from build123d import *

# Parameters (mm, degrees)
SKETCH2_W            = 230
SKETCH2_H            = 42
BOSS_EXTRUDE1_DEPTH  = 60
BOSS_EXTRUDE2_DEPTH  = 150
SKETCH5_R            = 4
CUT_EXTRUDE1_DEPTH   = 277
SKETCH7_R            = 4
BOSS_EXTRUDE3_DEPTH  = 20
SKETCH7_2_R          = 4
CUT_EXTRUDE2_DEPTH   = 10
SKETCH8_W            = 62
SKETCH8_H            = 24.6
BOSS_EXTRUDE4_DEPTH  = 14
SKETCH9_W            = 62
SKETCH9_H            = 24.6
BOSS_EXTRUDE5_DEPTH  = 14
SKETCH15_W           = 42
SKETCH15_H           = 60
SKETCH15_R           = 4
CUT_EXTRUDE3_DEPTH   = 5
SKETCH17_W           = 42
SKETCH17_H           = 60
SKETCH17_R           = 4
CUT_EXTRUDE4_DEPTH   = 5
SKETCH18_W           = 1
SKETCH18_H           = 62
BOSS_EXTRUDE9_DEPTH  = 24.6
SKETCH18_3_R         = 3
CUT_EXTRUDE5_DEPTH   = 35
SKETCH19_W           = 1
SKETCH19_H           = 62
BOSS_EXTRUDE10_DEPTH = 24.6
SKETCH19_3_R         = 3
CUT_EXTRUDE6_DEPTH   = 27
SKETCH20_W           = 15
SKETCH20_H           = 62
SKETCH20_R           = 3
BOSS_EXTRUDE11_DEPTH = 1
SKETCH21_W           = 15
SKETCH21_H           = 62
SKETCH21_R           = 3
BOSS_EXTRUDE12_DEPTH = 1
SKETCH23_W           = 255
SKETCH23_H           = 10
BOSS_EXTRUDE13_DEPTH = 150
SKETCH25_W           = 251.390716306
SKETCH25_H           = 22.262694164
CUT_EXTRUDE7_DEPTH   = 150
BOSS_EXTRUDE16_DEPTH = 17
CUT_EXTRUDE8_DEPTH   = 150
SKETCH28_W           = 255
SKETCH28_H           = 13
CUT_EXTRUDE9_DEPTH   = 167
BOSS_EXTRUDE18_DEPTH = 6
CUT_EXTRUDE10_DEPTH  = 43
SKETCH32_W           = 10
SKETCH32_H           = 20
BOSS_EXTRUDE19_DEPTH = 7.5
SKETCH33_W           = 10
SKETCH33_H           = 20
BOSS_EXTRUDE20_DEPTH = 8
SKETCH38_R           = 2.5
CUT_EXTRUDE12_DEPTH  = 16
SKETCH40_W           = 20.026518065
SKETCH40_H           = 12.666252083
CUT_EXTRUDE13_DEPTH  = 116
SKETCH41_W           = 84.423481935
SKETCH41_H           = 10
SKETCH41_W_2         = 110.05
BOSS_EXTRUDE21_DEPTH = 61.47
SKETCH42_W           = 10
SKETCH42_H           = 25
CUT_EXTRUDE14_DEPTH  = 10
SKETCH40_3_W         = 20
SKETCH40_3_H         = 10
BOSS_EXTRUDE22_DEPTH = 162.1
SKETCH43_W           = 10
SKETCH43_H           = 31.300449652
BOSS_EXTRUDE23_DEPTH = 40.5
BOSS_EXTRUDE24_START = -60
SKETCH46_W           = 20
SKETCH46_H           = 20
BOSS_EXTRUDE24_DEPTH = 222.1
SKETCH48_R           = 2
CUT_EXTRUDE15_DEPTH  = 30


with BuildPart() as part:
    # Sketch2 → Boss-Extrude1 (new body)
    with BuildSketch(Plane(origin=(0, 0, 0), x_dir=(1, 0, 0), z_dir=(0, 1, 0))):
        Polygon((-125, -31), (125, -31), (125, -21), (125, 0), (125, 21), (125, 31), (-125, 31), (-125, 21), (-125, 0), (-125, -21), align=None)
        Rectangle(SKETCH2_W, SKETCH2_H, mode=Mode.SUBTRACT)
    extrude(amount=BOSS_EXTRUDE1_DEPTH)

    # Sketch4 → Boss-Extrude2 (add)
    with BuildSketch(Plane.XZ):
        Polygon((125, 31), (-125, 31), (-125, 21), (-115, 21), (125, 21), align=None)
    extrude(amount=BOSS_EXTRUDE2_DEPTH)

    # Sketch5 → Cut-Extrude1 (cut)
    with BuildSketch(Plane.ZY.offset(125)):
        with Locations((0, 15.395589143)):
            Circle(SKETCH5_R)
        with Locations((0, 45.395589143)):
            Circle(SKETCH5_R)
    extrude(amount=-CUT_EXTRUDE1_DEPTH, mode=Mode.SUBTRACT)

    # Sketch7 → Boss-Extrude3 (add)
    with BuildSketch(Plane(origin=(125, 0, 0), x_dir=(0, 0, -1), z_dir=(1, 0, 0))):
        Polygon((-21, -150), (-31, -150), (-31, 60), (31, 60), (31, 0), (-21, 0), align=None)
        with Locations((0, 15.395589143)):
            Circle(SKETCH7_R, mode=Mode.SUBTRACT)
        with Locations((0, 45.395589143)):
            Circle(SKETCH7_R, mode=Mode.SUBTRACT)
    extrude(amount=-BOSS_EXTRUDE3_DEPTH)

    # Sketch7<2> → Cut-Extrude2 (cut)
    with BuildSketch(Plane(origin=(125, 0, 0), x_dir=(0, 0, -1), z_dir=(1, 0, 0))):
        Polygon((-21, -150), (-31, -150), (-31, 60), (31, 60), (31, 0), (-21, 0), align=None)
        with Locations((0, 15.395589143)):
            Circle(SKETCH7_2_R, mode=Mode.SUBTRACT)
        with Locations((0, 45.395589143)):
            Circle(SKETCH7_2_R, mode=Mode.SUBTRACT)
    extrude(amount=-CUT_EXTRUDE2_DEPTH, mode=Mode.SUBTRACT)

    # Sketch8 → Boss-Extrude4 (add)
    with BuildSketch(Plane(origin=(115, 0, 0), x_dir=(0, 0, -1), z_dir=(1, 0, 0))):
        with Locations((0, 12.3)):
            Rectangle(SKETCH8_W, SKETCH8_H)
    extrude(amount=BOSS_EXTRUDE4_DEPTH)

    # Sketch9 → Boss-Extrude5 (add)
    with BuildSketch(Plane.ZY.offset(125)):
        with Locations((0, 47.7)):
            Rectangle(SKETCH9_W, SKETCH9_H)
    extrude(amount=BOSS_EXTRUDE5_DEPTH)

    # Sketch15 → Cut-Extrude3 (cut)
    with BuildSketch(Plane.ZY.offset(-105)):
        with Locations((0, 30)):
            Rectangle(SKETCH15_W, SKETCH15_H)
        with Locations((0, 15.395589143)):
            Circle(SKETCH15_R, mode=Mode.SUBTRACT)
        with Locations((0, 45.395589143)):
            Circle(SKETCH15_R, mode=Mode.SUBTRACT)
    extrude(amount=-CUT_EXTRUDE3_DEPTH, mode=Mode.SUBTRACT)

    # Sketch17 → Cut-Extrude4 (cut)
    with BuildSketch(Plane(origin=(-115, 0, 0), x_dir=(0, 0, -1), z_dir=(1, 0, 0))):
        with Locations((0, 30)):
            Rectangle(SKETCH17_W, SKETCH17_H)
        with Locations((0, 45.395589143)):
            Circle(SKETCH17_R, mode=Mode.SUBTRACT)
        with Locations((0, 15.395589143)):
            Circle(SKETCH17_R, mode=Mode.SUBTRACT)
    extrude(amount=-CUT_EXTRUDE4_DEPTH, mode=Mode.SUBTRACT)

    # Sketch18 → Boss-Extrude9 (add)
    with BuildSketch(Plane.XZ.offset(-35.4)):
        with Locations((-139.5, 0)):
            Rectangle(SKETCH18_W, SKETCH18_H)
    extrude(amount=-BOSS_EXTRUDE9_DEPTH)

    # Sketch18<3> → Cut-Extrude5 (cut)
    with BuildSketch(Plane.XZ.offset(-35.4)):
        with Locations((-132.5, 21)):
            Circle(SKETCH18_3_R)
        with Locations((-132.5, -21)):
            Circle(SKETCH18_3_R)
    extrude(amount=-CUT_EXTRUDE5_DEPTH, mode=Mode.SUBTRACT)

    # Sketch19 → Boss-Extrude10 (add)
    with BuildSketch(Plane(origin=(0, 24.6, 0), x_dir=(1, 0, 0), z_dir=(0, 1, 0))):
        with Locations((129.5, 0)):
            Rectangle(SKETCH19_W, SKETCH19_H)
    extrude(amount=-BOSS_EXTRUDE10_DEPTH)

    # Sketch19<3> → Cut-Extrude6 (cut)
    with BuildSketch(Plane(origin=(0, 24.6, 0), x_dir=(1, 0, 0), z_dir=(0, 1, 0))):
        with Locations((122.5, 21)):
            Circle(SKETCH19_3_R)
        with Locations((122.5, -21)):
            Circle(SKETCH19_3_R)
    extrude(amount=-CUT_EXTRUDE6_DEPTH, mode=Mode.SUBTRACT)

    # Sketch20 → Boss-Extrude11 (add)
    with BuildSketch(Plane(origin=(0, 24.6, 0), x_dir=(1, 0, 0), z_dir=(0, 1, 0))):
        with Locations((122.5, 0)):
            Rectangle(SKETCH20_W, SKETCH20_H)
        with Locations((122.5, -21)):
            Circle(SKETCH20_R, mode=Mode.SUBTRACT)
        with Locations((122.5, 21)):
            Circle(SKETCH20_R, mode=Mode.SUBTRACT)
    extrude(amount=BOSS_EXTRUDE11_DEPTH)

    # Sketch21 → Boss-Extrude12 (add)
    with BuildSketch(Plane.XZ.offset(-35.4)):
        with Locations((-132.5, 0)):
            Rectangle(SKETCH21_W, SKETCH21_H)
        with Locations((-132.5, 21)):
            Circle(SKETCH21_R, mode=Mode.SUBTRACT)
        with Locations((-132.5, -21)):
            Circle(SKETCH21_R, mode=Mode.SUBTRACT)
    extrude(amount=BOSS_EXTRUDE12_DEPTH)

    # Sketch23 → Boss-Extrude13 (add)
    with BuildSketch(Plane.XZ):
        with Locations((2.5, -26)):
            Rectangle(SKETCH23_W, SKETCH23_H)
    extrude(amount=BOSS_EXTRUDE13_DEPTH)

    # Sketch25 → Cut-Extrude7 (cut)
    with BuildSketch(Plane.XZ):
        with Locations((-4.583562675, 27.327499947)):
            Rectangle(SKETCH25_W, SKETCH25_H)
    extrude(amount=CUT_EXTRUDE7_DEPTH, mode=Mode.SUBTRACT)

    # Sketch26 → Boss-Extrude16 (add)
    with BuildSketch(Plane(origin=(0, 0, -31), x_dir=(-1, 0, 0), z_dir=(0, 0, -1))):
        Polygon((125, -150), (-130, -150), (-130, 25.6), (-115, 25.6), (-115, 60), (125, 60), (140, 60), (140, 34.4), (125, 34.4), (125, 25.6), align=None)
    extrude(amount=BOSS_EXTRUDE16_DEPTH)

    # Sketch27 → Cut-Extrude8 (cut)
    with BuildSketch(Plane.XZ):
        Polygon((110, -31), (132.347433228, -31), (132.347433228, -21), (110, -21), (-153.412168614, -21), (-153.412168614, -31), align=None)
    extrude(amount=CUT_EXTRUDE8_DEPTH, mode=Mode.SUBTRACT)

    # Sketch28 → Cut-Extrude9 (cut)
    with BuildSketch(Plane.XZ):
        with Locations((2.5, -37.5)):
            Rectangle(SKETCH28_W, SKETCH28_H)
    extrude(amount=CUT_EXTRUDE9_DEPTH, mode=Mode.SUBTRACT)

    # Sketch29 → Boss-Extrude18 (add)
    with BuildSketch(Plane(origin=(0, 0, -48), x_dir=(-1, 0, 0), z_dir=(0, 0, -1))):
        Polygon((125, -150), (-130, -150), (-130, 25.6), (-115, 25.6), (-115, 60), (125, 60), (140, 60), (140, 34.4), (125, 34.4), (125, 25.6), align=None)
    extrude(amount=BOSS_EXTRUDE18_DEPTH)

    # Sketch31 → Cut-Extrude10 (cut)
    with BuildSketch(Plane.XY.offset(-44)):
        Polygon((33.05, -150), (130, -150), (130, -100.63), (33.05, -100.63), (33.05, -80.63), (-22.95, -80.63), (-22.95, -100.63), (-125, -100.63), (-125, -150), align=None)
    extrude(amount=-CUT_EXTRUDE10_DEPTH, mode=Mode.SUBTRACT)

    # Sketch32 → Boss-Extrude19 (add)
    with BuildSketch(Plane.ZY.offset(-33.05)):
        with Locations((-49, -90.63)):
            Rectangle(SKETCH32_W, SKETCH32_H)
    extrude(amount=BOSS_EXTRUDE19_DEPTH)

    # Sketch33 → Boss-Extrude20 (add)
    with BuildSketch(Plane(origin=(-22.95, 0, 0), x_dir=(0, 0, -1), z_dir=(1, 0, 0))):
        with Locations((49, -90.63)):
            Rectangle(SKETCH33_W, SKETCH33_H)
    extrude(amount=BOSS_EXTRUDE20_DEPTH)

    # Sketch38 → Cut-Extrude12 (cut)
    with BuildSketch(Plane.XY.offset(-44)):
        with Locations((29.35, -95.53)):
            Circle(SKETCH38_R)
        with Locations((29.35, -85.73)):
            Circle(SKETCH38_R)
        with Locations((-19.25, -95.53)):
            Circle(SKETCH38_R)
        with Locations((-19.25, -85.73)):
            Circle(SKETCH38_R)
    extrude(amount=-CUT_EXTRUDE12_DEPTH, mode=Mode.SUBTRACT)

    # Sketch40 → Cut-Extrude13 (cut)
    with BuildSketch(Plane.XZ):
        with Locations((119.986740967, -50.333126042)):
            Rectangle(SKETCH40_W, SKETCH40_H)
    extrude(amount=CUT_EXTRUDE13_DEPTH, mode=Mode.SUBTRACT)

    # Sketch41 → Boss-Extrude21 (add)
    with BuildSketch(Plane.XZ.offset(100.63)):
        with Locations((67.761740968, -49)):
            Rectangle(SKETCH41_W, SKETCH41_H)
        with Locations((-69.975, -49)):
            Rectangle(SKETCH41_W_2, SKETCH41_H)
    extrude(amount=BOSS_EXTRUDE21_DEPTH)

    # Sketch42 → Cut-Extrude14 (cut)
    with BuildSketch(Plane.ZY.offset(-25.55)):
        with Locations((-49, -118.299550348)):
            Rectangle(SKETCH42_W, SKETCH42_H)
    cut_extrude14 = extrude(amount=-CUT_EXTRUDE14_DEPTH, mode=Mode.SUBTRACT)

    # Mirror1: Cut-Extrude14 across plane
    add(cut_extrude14.mirror(Plane.ZY.offset(-5.3)), mode=Mode.SUBTRACT)

    # Sketch40<3> → Boss-Extrude22 (add)
    with BuildSketch(Plane.XZ):
        with Locations((79.973481935, -39)):
            Rectangle(SKETCH40_3_W, SKETCH40_3_H)
        with Locations((-89.973481935, -39)):
            Rectangle(SKETCH40_3_W, SKETCH40_3_H)
    extrude(amount=BOSS_EXTRUDE22_DEPTH)

    # Sketch43 → Boss-Extrude23 (add)
    with BuildSketch(Plane.ZY.offset(-25.55)):
        with Locations((-49, -146.449775174)):
            Rectangle(SKETCH43_W, SKETCH43_H)
    extrude(amount=BOSS_EXTRUDE23_DEPTH)

    # Sketch46 → Boss-Extrude24 (add)
    with BuildSketch(Plane.XZ.offset(BOSS_EXTRUDE24_START)):
        with Locations((79.973481935, 31)):
            Rectangle(SKETCH46_W, SKETCH46_H)
        with Locations((-89.973481935, 31)):
            Rectangle(SKETCH46_W, SKETCH46_H)
    extrude(amount=BOSS_EXTRUDE24_DEPTH)

    # Sketch48 → Cut-Extrude15 (cut)
    with BuildSketch(Plane.XZ.offset(162.1)):
        with Locations((79.973481935, 31)):
            Circle(SKETCH48_R)
        with Locations((79.973481935, -44)):
            Circle(SKETCH48_R)
        with Locations((-89.973481935, 31)):
            Circle(SKETCH48_R)
        with Locations((-89.973481935, -44)):
            Circle(SKETCH48_R)
    extrude(amount=-CUT_EXTRUDE15_DEPTH, mode=Mode.SUBTRACT)


solid = part.part
Geometry: final body of the model. Coordinates: model frame, mm. A direction names the side the tool comes from. Round coordinates to 2 decimals unless told otherwise and drop trailing zeros. Loops run counter-clockwise (first coordinate to the right, second up) from the corner with the lowest first, then second, coordinate; pieces in that order, holes last.
Q1. Pin query (flat end, axial travel): P1, Ø8, axis at x = -19.25, y = -85.73, coming from the +Z side; P2, Ø5, axis at y = -65, z = -49, coming from the +X side; P3, Ø2, axis at x = 79.5, z = -44, coming from the -Y side. Return the tip coordinate at first contact, or that it passes through.
Q2. Access query for faces 4 (the flat face through (-6, 0, 26)), 5 (the flat face through (-133, 34.4, -11)), 6 (the flat face through (109.973, -80, -49)). Directions: +Z, -Z, +X, -X, +Y, -Y. A direction counts if a zero-diameter tool reaches every point of the face in a straight line with its end or side. Return the directions, or none.
Q3. Section D-D on z = 12. Return loops of the section in (x, y), plus the area to 3 significant figures.
Q4. Section A-A on y = -146. Return loops of the section in (x, z), plus the area to 3 significant figures.
Q5. Pull-direction query (Z, two-part tool) for faces 1 (the flat face through (-14.95, -93, -49)), 2 (the flat face through (-125, 45, 0)), 3 (the flat face through (105, 30, 31)); classes: released by +Z, released by -Z, zero draft, split by the parting line, or undercut.
Q6. Material intervals for L1, parallel to Y at x = 111.65, z = 0; L2, parallel to Z at x = -132.5, y = 46.5; L3, parallel to Z at x = 59.5, y = 26.5, sorted ascending.
Q7. Section B-B on x = 16. Return loops of the section in (y, z), plus the area to 3 significant figures.
Q8. Section C-C on y = 3. Return loops of the section in (x, z).
Evaluation:
1. P1: stops at z = -44
1. P2: stops at x = 109.97
1. P3: stops at y = -132.1
2. face 4: +Z, -Y
2. face 5: +Z, -Z, -X, -Y
2. face 6: +Z, -Z, +X, -Y
3. outline: (-140, 34.4) - (-125, 34.4) - (-125, 0) - (-120, 0) - (-120, 60) - (-140, 60) - close; (110, 0) - (130, 0) - (130, 25.6) - (115, 25.6) - (115, 60) - (110, 60) - close
3. area: 1,370 mm2
4. outline: (-125, -54) - (109.97, -54) - (109.97, -44) - (89.97, -44) - (89.97, -34) - (69.97, -34) - (69.97, -44) - (-79.97, -44) - (-79.97, -34) - (-99.97, -34) - (-99.97, -44) - (-125, -44) - close; (-99.97, 21) - (-79.97, 21) - (-79.97, 41) - (-99.97, 41) - close; (69.97, 21) - (89.97, 21) - (89.97, 41) - (69.97, 41) - close; hole circle Ø4 at (-89.97, -44); hole circle Ø4 at (-89.97, 31); hole circle Ø4 at (79.97, -44); hole circle Ø4 at (79.97, 31)
4. area: 3,500 mm2
5. face 1: zero draft
5. face 2: undercut
5. face 3: released by +Z
6. L1: y = 0 to 11.4, 19.4 to 41.4, 49.4 to 60
6. L2: z = -54 to -24, -18 to 18, 24 to 31
6. L3: z = -54 to -21, 21 to 31
7. outline: (-162.1, -54) - (-130.8, -54) - (-130.8, -44) - (-162.1, -44) - close; (-80.63, -54) - (60, -54) - (60, -21) - (0, -21) - (0, -44) - (-80.63, -44) - close; (0, 21) - (60, 21) - (60, 31) - (0, 31) - close
7. area: 3,700 mm2
8. outline: (-125, -54) - (130, -54) - (130, 31) - (89.97, 31) - (89.97, 41) - (69.97, 41) - (69.97, 31) - (-79.97, 31) - (-79.97, 41) - (-99.97, 41) - (-99.97, 31) - (-125, 31) - close; hole (-120, -21) - (110, -21) - (110, 21) - (-120, 21) - close; hole circle Ø6 at (122.5, -21); hole circle Ø6 at (122.5, 21)
